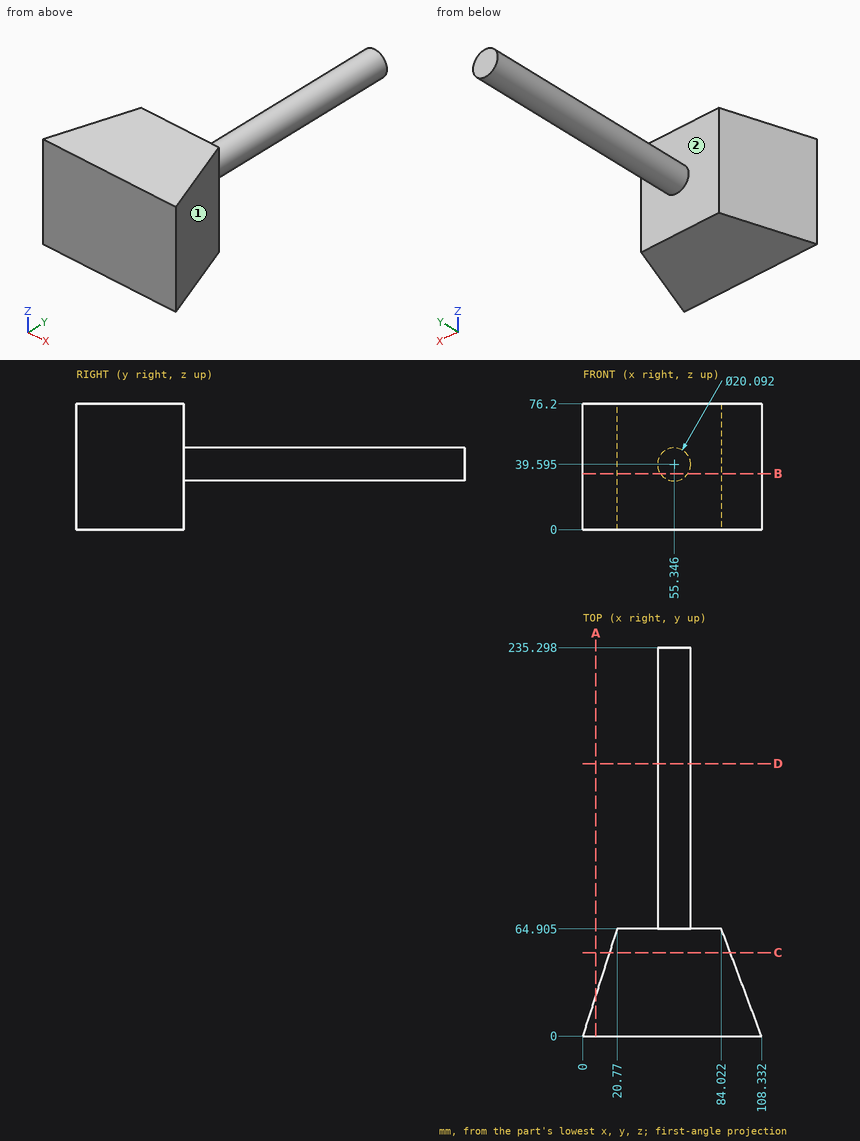
Answer from the drawing. Dimensions are ordinates in mm from the lowest x, y and z of the part. A direction names the side the tool comes from. Coordinates: 2 decimals unless noted, no trailing zeros. Order: outer loops, then holes, each group sorted by start corner. A loop starts at its lowest first (then second) coordinate and runs counter-clockwise, first axis right, second up. Notation, with made-up numbers: M 89,-36 L 142,-36 A19 ccw 142,-25 Z; hole C 82,13 d5. An arc over 180 degrees is marked long. Put each result on its own line as item: value. Start each with the question number.
Item 1: Section B-B, the plane z = 34 is taken. Determine the outline of the cut face in (x, y) (1 decimal), plus the area to 3 significant figures.
Item 2: For the marked faces 1 and 2, determine the directions among +Z, -Z, +X, -X, +Y, -Y from which every point of the face is accessible in a straight line to the end or side of a thin tool.
Item 3: Given pin 1 Ø10 at (y, z) = (36.5, 32.5) entering from +X; pin 2 Ø4 at (x, z) = (72, 67) entering from +Y (1 decimal), each flat-ended and moving along its own axis, determine where each tip first touches the part or whether it passes through.
Item 4: Section C-C, the plane y = 50.5 is taken. Determine the outline of the cut face in (x, z).
Item 5: Section D-D, the plane y = 165 is taken. Determine the outline of the cut face in (x, z) (1 decimal).
Item 6: Consider probe 1 along Y at (x, z) = (78.5, 45.5) (1 decimal); probe 2 along X at (y, z) = (46, 10); probe 3 along X at (y, z) = (135, 39) (1 decimal). Determine where each line is inside the solid, lowest interval first. Write a range as [from, to].
Item 7: Section A-A, the plane x = 8 is taken. Determine the outline of the cut face in (y, z).
Computed:
1. outline: M 0,0 L 108.3,0 L 84,64.9 L 63.7,64.9 L 63.7,235.3 L 47,235.3 L 47,64.9 L 20.8,64.9 Z
1. area: 8,410 mm2
2. face 1: +Z, -Z, +X, +Y
2. face 2: +Y
3. pin 1: stops at x = 96.53
3. pin 2: stops at y = 64.9
4. outline: M 16.16,0 L 89.42,0 L 89.42,76.2 L 16.16,76.2 Z
5. outline: C 55.3,39.6 d20.1
6. probe 1: y = [0, 64.9]
6. probe 2: x = [14.72, 91.1]
6. probe 3: x = [45.3, 65.4]
7. outline: M 0,0 L 25,0 L 25,76.2 L 0,76.2 Z
